The listing builds one solid part. Answer for the finished solid, in the listing's coordinates (mm). Face numbers are marked on the shaded views. A direction names the side the tool comes from. Coordinates: 2 decimals unless noted, no trailing zeros. Write each loop counter-clockwise with the first axis right and the second up, starting at its lowest first coordinate (ties: lowest second). Pieces come first, ordered by that corner, then holes.
from build123d import *

# Parameters (mm, degrees)
SKETCH36_R          = 0.6
SIDE_HOLES_DEPTH    = 2
CIRPATTERN2_COUNT   = 2
SKETCH38_W          = 1.525968236
SKETCH38_H          = 25
BOSS_EXTRUDE5_DEPTH = 1.25
BOSS_EXTRUDE6_DEPTH = 0.5
CIRPATTERN3_COUNT   = 3
SKETCH39_R          = 22
SKETCH39_R_2        = 12.63
BOSS_EXTRUDE7_DEPTH = 1.5
SKETCH40_R          = 0.6
CUT_EXTRUDE1_DEPTH  = 48.734856834
CIRPATTERN4_COUNT   = 3
BOSS_EXTRUDE8_START = 1
SKETCH41_R          = 13.545580942
SKETCH41_R_2        = 12.63
BOSS_EXTRUDE8_DEPTH = 1
SKETCH42_R          = 13.545580942
SKETCH42_R_2        = 12.63
BOSS_EXTRUDE9_DEPTH = 1


with BuildPart() as part:
    # Sketch35 → Revolve1 (revolve)
    with BuildSketch(Plane.XY, mode=Mode.PRIVATE) as revolve1_sk:
        Polygon((20.474031764, 11.202438329), (12.63, 0), (14.155968236, 0), (22, 11.202438329), align=None)
    revolve(revolve1_sk.sketch.rotate(Axis((0, 11.202438329, 0), (0, -1, 0)), 90), axis=Axis((0, 11.202438329, 0), (0, -1, 0)))

    # Sketch36 → side-holes (cut, symmetric)
    with BuildSketch(Plane(origin=(8.474857205, -5.9341589, 0), x_dir=(0, 0, 1), z_dir=(-0.8191520442889934, 0.5735764363510439, 0))):
        with Locations(Location((0, 18.744270391, 0), (0, 0, 239.229798776))):
            Circle(SKETCH36_R)
    side_holes = extrude(amount=SIDE_HOLES_DEPTH, both=True, mode=Mode.SUBTRACT)

    # CirPattern2: side-holes ×2 about axis
    cirpattern2_axis = Axis((0, 0, 0), (0, 1, 0))
    for i in range(1, CIRPATTERN2_COUNT):
        add(side_holes.rotate(cirpattern2_axis, i * 360 / CIRPATTERN2_COUNT), mode=Mode.SUBTRACT)

    # Sketch38 → Boss-Extrude5 (add, symmetric)
    with BuildSketch(Plane(origin=(0, 0, 0), x_dir=(0, 0, -1), z_dir=(1, 0, 0))):
        with Locations((13.392984118, -12.5)):
            Rectangle(SKETCH38_W, SKETCH38_H)
    boss_extrude5 = extrude(amount=BOSS_EXTRUDE5_DEPTH, both=True)

    # Sketch38<6> → Boss-Extrude6 (add, symmetric)
    with BuildSketch(Plane(origin=(0, 0, 0), x_dir=(0, 0, -1), z_dir=(1, 0, 0))):
        Polygon((19.63, 9.997036047), (12.63, 0), (14.155968236, 0), (14.155968236, -25), (21.155968236, -25), (21.155968236, 9.997036047), align=None)
    boss_extrude6 = extrude(amount=BOSS_EXTRUDE6_DEPTH, both=True)

    # CirPattern3: Boss-Extrude5, Boss-Extrude6 ×3 about axis
    cirpattern3_axis = Axis((0, 0, 0), (0, 1, 0))
    add([boss_extrude5.rotate(cirpattern3_axis, i * 360 / CIRPATTERN3_COUNT) for i in range(1, CIRPATTERN3_COUNT)])
    add([boss_extrude6.rotate(cirpattern3_axis, i * 360 / CIRPATTERN3_COUNT) for i in range(1, CIRPATTERN3_COUNT)])

    # Sketch39 → Boss-Extrude7 (add)
    with BuildSketch(Plane.XZ.offset(25)):
        with Locations(Location((0, 0, 0), (0, 0, 270))):
            Circle(SKETCH39_R)
        with Locations(Location((0, 0, 0), (0, 0, 270))):
            Circle(SKETCH39_R_2, mode=Mode.SUBTRACT)
    extrude(amount=BOSS_EXTRUDE7_DEPTH)

    # Sketch40 → Cut-Extrude1 (cut, through all)
    with BuildSketch(Plane(origin=(0, -25, 0), x_dir=(1, 0, 0), z_dir=(0, 1, 0))):
        with Locations(Location((0, -17.315, 0), (0, 0, 270))):
            Circle(SKETCH40_R)
    cut_extrude1 = extrude(amount=-CUT_EXTRUDE1_DEPTH, mode=Mode.SUBTRACT)

    # CirPattern4: Cut-Extrude1 ×3 about axis
    cirpattern4_axis = Axis((0, 0, 0), (0, 1, 0))
    for i in range(1, CIRPATTERN4_COUNT):
        add(cut_extrude1.rotate(cirpattern4_axis, i * 360 / CIRPATTERN4_COUNT), mode=Mode.SUBTRACT)

    # Sketch41 → Boss-Extrude8 (add)
    with BuildSketch(Plane(origin=(0, -25, 0), x_dir=(1, 0, 0), z_dir=(0, 1, 0)).offset(BOSS_EXTRUDE8_START)):
        Circle(SKETCH41_R)
        with Locations(Location((0, 0, 0), (0, 0, 90))):
            Circle(SKETCH41_R_2, mode=Mode.SUBTRACT)
    extrude(amount=-BOSS_EXTRUDE8_DEPTH)

    # Sketch42 → Boss-Extrude9 (add)
    with BuildSketch(Plane.XZ):
        Circle(SKETCH42_R)
        with Locations(Location((0, 0, 0), (0, 0, 270))):
            Circle(SKETCH42_R_2, mode=Mode.SUBTRACT)
    extrude(amount=BOSS_EXTRUDE9_DEPTH)


solid = part.part
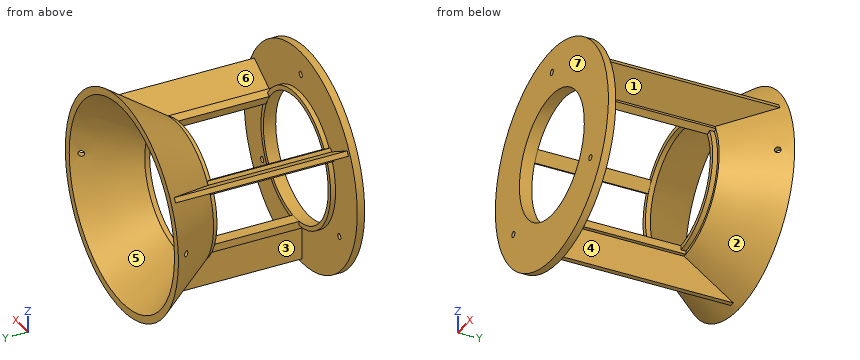
Q1. The part is cut by section A-A, the plane y = -17. Write down the section's boundary in (x, z), then the cut area to 3 significant figures.
Answers below:
outline: (-18.57, 10.14) - (-12.51, 6.64) - (-12.88, 6) - (-11.56, 5.23) - (-10.31, 7.4) - (-11.63, 8.16) - (-12.01, 7.51) - (-18.07, 11.01) - close; (-1.25, -14.16) - (-0.5, -14.16) - (-0.5, -21.16) - (0.5, -21.16) - (0.5, -14.16) - (1.25, -14.16) - (1.25, -12.63) - (-1.25, -12.63) - close; (10.31, 7.4) - (11.56, 5.23) - (12.88, 6) - (12.51, 6.64) - (18.57, 10.14) - (18.07, 11.01) - (12.01, 7.51) - (11.63, 8.16) - close
area: 32.4 mm2
Q2. The part is cut by section B-B, the plane z = -5.5. State how many separate pieces and enclosed holes the cut face has, then the cut area to 3 significant figures.
Answers below:
separate pieces: 4
enclosed holes: 0
area: 70.0 mm2
Q3. Find the intervals of material crossed by probe 1 along Y at (x, z) = (18, 11); probe 2 along X at (y, z) = (-4, 8); probe 3 along X at (y, z) = (-5.5, -13), in increasing order.
Answers below:
probe 1: y = -26.5 to -25, 9.91 to 11.2
probe 2: x = -14.86 to -12.86, -11.73 to -11.36, 11.36 to 11.73, 12.86 to 14.86
probe 3: x = -1.25 to 1.25
Q4. Given pin 1 (1.5 mm diameter, centred on x = 9.5, z = -13, fed in from +Y); pin 2 (0.8 mm diameter, centred on y = -14, z = -13.5, fed in from +X); pin 3 (6 mm diameter, centred on x = -3.5, z = -14.5, fed in from +Y); pin 4 (4 mm diameter, centred on x = -8, z = -8, fed in from -Y), each flat-ended and moving along its own axis, determine where each tip first touches the part or whether it passes through.
Answers below:
pin 1: stops at y = 6.03
pin 2: stops at x = 1.25
pin 3: stops at y = 7.55
pin 4: stops at y = -26.5
Q5. Which of the six approach directions +Z, -Z, +X, -X, +Y, -Y give full straight-line access (tool end or side, diameter ignored) to the marked faces 1, 2, 3 and 4?
Answers below:
face 1: +X
face 2: none
face 3: -Z, -X
face 4: -Z, +X
Q6. Determine the mould class of the marked faces 5, 6 and 7 for opening direction Z: released by +Z, released by -Z, zero draft, split by the parting line, or undercut.
Answers below:
face 5: undercut
face 6: released by +Z
face 7: zero draft
